The drawing under review shows one solid part. Ordinate dimensions are in mm from its lowest x, y, z. A direction names the side the tool comes from. Give positions to 0.01 mm unless a question says otherwise; leave off trailing zeros. Loops run counter-clockwise (first coordinate to the right, second up) from the corner with the lowest first, then second, coordinate; pieces in that order, holes last.
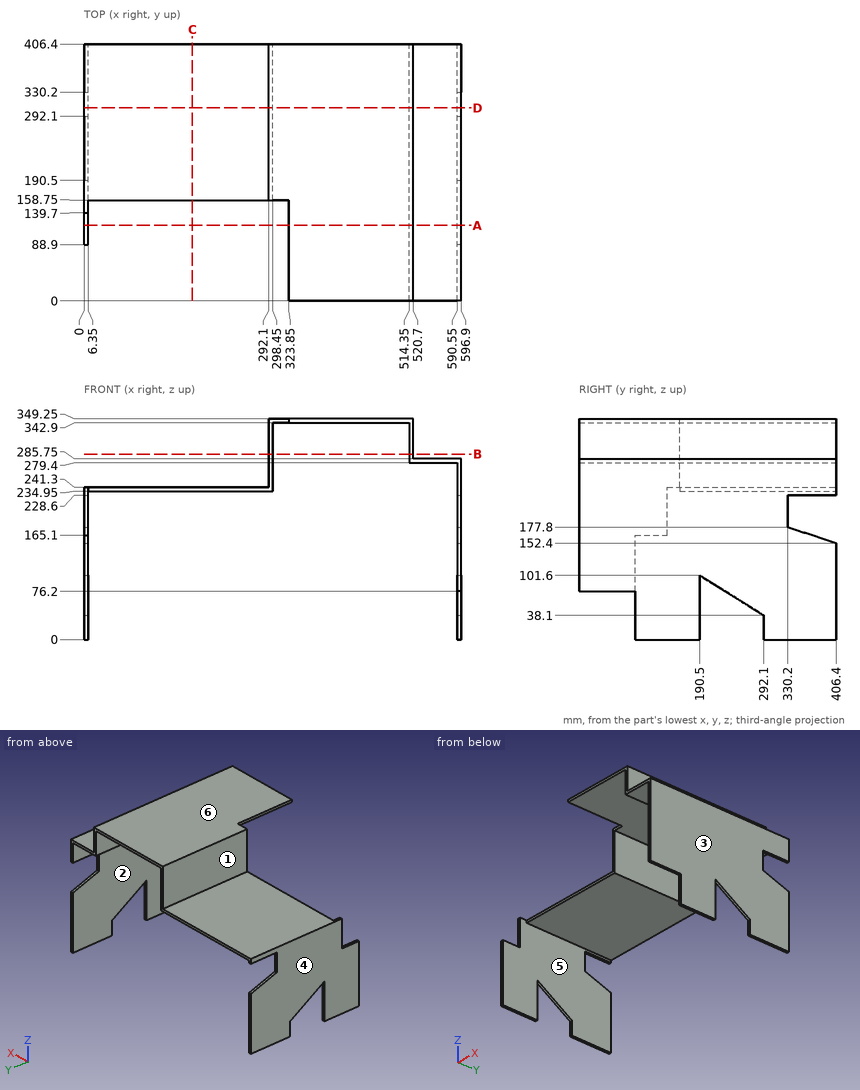
Item 1: Take a section at D-D on y = 305.5. Give the boundary of the cut face in (x, z).
Answer:
outline: (0, 0) - (6.35, 0) - (6.35, 234.95) - (298.45, 234.95) - (298.45, 342.9) - (514.35, 342.9) - (514.35, 279.4) - (590.55, 279.4) - (590.55, 0) - (596.9, 0) - (596.9, 285.75) - (520.7, 285.75) - (520.7, 349.25) - (292.1, 349.25) - (292.1, 241.3) - (0, 241.3) - close
Item 2: Clearance check with flat-ended pins moving along their axes: pin 1 Ø5 at (y, z) = (306, 202.5) entering from -X; pin 2 Ø3 at (x, y) = (249, 314.5) entering from +Z; pin 3 Ø8 at (x, y) = (238.5, 308.5) entering from -Z; pin 4 Ø1.9 at (x, z) = (2.5, 194.5) entering from +Y. State where each tip first meets the part, or that it passes through.
Answer:
pin 1: stops at x = 0
pin 2: stops at z = 241.3
pin 3: stops at z = 234.95
pin 4: stops at y = 330.2
Item 3: Take a section at B-B on z = 293.5. Give the boundary of the cut face in (x, y), and give its area (3 significant figures).
Answer:
outline: (292.1, 158.75) - (298.45, 158.75) - (298.45, 406.4) - (292.1, 406.4) - close; (514.35, 0) - (520.7, 0) - (520.7, 406.4) - (514.35, 406.4) - close
area: 4,150 mm2
Item 4: Take a section at A-A on y = 119.5. Give the boundary of the cut face in (x, z).
Answer:
outline: (0, 0) - (6.35, 0) - (6.35, 165.1) - (0, 165.1) - close; (323.85, 342.9) - (514.35, 342.9) - (514.35, 279.4) - (590.55, 279.4) - (590.55, 0) - (596.9, 0) - (596.9, 285.75) - (520.7, 285.75) - (520.7, 349.25) - (323.85, 349.25) - close
Item 5: For L1, parallel to X at y = 301.5, z = 153; L2, parallel to Z at x = 43.5, y = 371; L3, parallel to Z at x = 335, y = 361, list the stretches that pass through material, from the lowest coordinate up.
Answer:
L1: x = 0 to 6.35, 590.55 to 596.9
L2: z = 234.95 to 241.3
L3: z = 342.9 to 349.25
Item 6: The part is to be moulded in two halves that separate along X. For the marked faces 4, 5 and 6, say which applies: released by +X, released by -X, zero draft, split by the parting line, or undercut.
Answer:
face 4: released by -X
face 5: undercut
face 6: zero draft
Item 7: Tool access review of the marked faces 1, 2 and 3: name each direction out of +Z, -Z, +X, -X, +Y, -Y from which nothing blocks a thin tool from reaching the whole face with its end or side.
Answer:
face 1: +Z, -X, +Y, -Y
face 2: -Z, +Y, -Y
face 3: +Z, -Z, +X, +Y, -Y
Item 8: Take a section at C-C on x = 171.5. Give the boundary of the cut face in (y, z).
Answer:
outline: (158.75, 234.95) - (406.4, 234.95) - (406.4, 241.3) - (158.75, 241.3) - close
